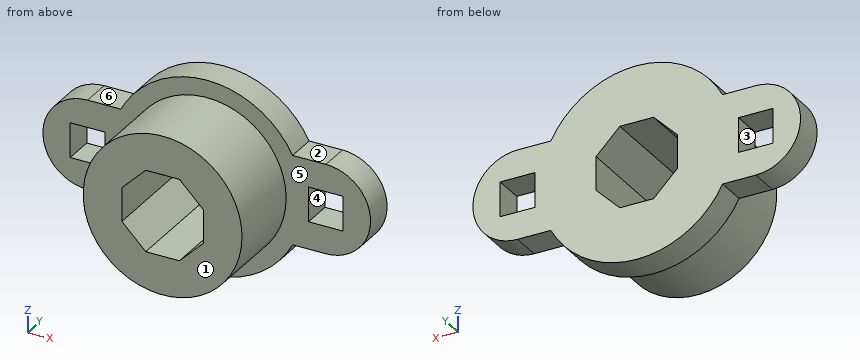
from build123d import *

# Parameters (mm, degrees)
SKETCH1_R           = 8
BOSS_EXTRUDE1_DEPTH = 8
SKETCH2_R           = 9.75
BOSS_EXTRUDE2_DEPTH = 3
BOSS_EXTRUDE3_DEPTH = 3
CUT_EXTRUDE2_REACH  = 13
SKETCH5_W           = 3.5
SKETCH5_H           = 3.5
CUT_EXTRUDE1_DEPTH  = 12


with BuildPart() as part:
    # Sketch1 → Boss-Extrude1 (new body)
    with BuildSketch(Plane(origin=(0, 0, 0), x_dir=(1, 0, 0), z_dir=(0, 1, 0))):
        Circle(SKETCH1_R)
    extrude(amount=BOSS_EXTRUDE1_DEPTH)

    # Sketch2 → Boss-Extrude2 (add)
    with BuildSketch(Plane(origin=(0, 8, 0), x_dir=(1, 0, 0), z_dir=(0, 1, 0))):
        Circle(SKETCH2_R)
    extrude(amount=BOSS_EXTRUDE2_DEPTH)

    # Sketch4 → Boss-Extrude3 (add)
    with BuildSketch(Plane(origin=(0, 11, 0), x_dir=(1, 0, 0), z_dir=(0, 1, 0))):
        with BuildLine():
            Line((12, -4.5), (-12, -4.5))
            ThreePointArc((-12, -4.5), (-16.5, 0), (-12, 4.5))
            Line((-12, 4.5), (12, 4.5))
            ThreePointArc((12, 4.5), (16.5, 0), (12, -4.5))
        make_face()
    extrude(amount=-BOSS_EXTRUDE3_DEPTH)

    # Sketch5 → Cut-Extrude2 (cut, up to next)
    with BuildSketch(Plane(origin=(0, 11, 0), x_dir=(1, 0, 0), z_dir=(0, 1, 0)), mode=Mode.PRIVATE) as cut_extrude2_sk1:
        with Locations((-12, 0)):
            Rectangle(SKETCH5_W, SKETCH5_H)
    cut_extrude2_tool1 = extrude(cut_extrude2_sk1.sketch, amount=-CUT_EXTRUDE2_REACH, mode=Mode.PRIVATE) & part.part
    add(cut_extrude2_tool1.solids().sort_by_distance((-12, 11, 0))[0], mode=Mode.SUBTRACT)
    # Sketch5 → Cut-Extrude2 (cut, up to next)
    with BuildSketch(Plane(origin=(0, 11, 0), x_dir=(1, 0, 0), z_dir=(0, 1, 0)), mode=Mode.PRIVATE) as cut_extrude2_sk2:
        with Locations((12, 0)):
            Rectangle(SKETCH5_W, SKETCH5_H)
    cut_extrude2_tool2 = extrude(cut_extrude2_sk2.sketch, amount=-CUT_EXTRUDE2_REACH, mode=Mode.PRIVATE) & part.part
    add(cut_extrude2_tool2.solids().sort_by_distance((12, 11, 0))[0], mode=Mode.SUBTRACT)

    # Sketch3 → Cut-Extrude1 (cut, through all)
    with BuildSketch(Plane(origin=(0, 11, 0), x_dir=(1, 0, 0), z_dir=(0, 1, 0))):
        Polygon((4.1, 1.698275606), (1.698275606, 4.1), (-1.698275606, 4.1), (-4.1, 1.698275606), (-4.1, -1.698275606), (-1.698275606, -4.1), (1.698275606, -4.1), (4.1, -1.698275606), align=None)
    extrude(amount=-CUT_EXTRUDE1_DEPTH, mode=Mode.SUBTRACT)


solid = part.part
The listing builds one solid part. Answer for the finished solid, in the listing's coordinates (mm). Face numbers are marked on the shaded views. A direction names the side the tool comes from. Round coordinates to 2 decimals unless told otherwise and drop trailing zeros. Order: outer loops, then holes, each group sorted by start corner. A loop starts at its lowest first (then second) coordinate and runs counter-clockwise, first axis right, second up. Notation, with made-up numbers: (54.5, 74) -> (77.5, 74) arc R29 cw to (77.5, 111) -> close; hole circle Ø11 at (26.25, 44.5). An arc over 180 degrees is marked (long way). Write each question's results on one line, items separated by ' | '. Start each with the question number.
Q1. Which of the six approach directions +Z, -Z, +X, -X, +Y, -Y give full straight-line access (tool end or side, diameter ignored) to the marked faces 4, 5 and 6?
Q2. The mould has two halves that part along Z. Classify the marked faces 1, 2 and 3: pulls with the +Z half, pulls with the -Z half, needs draft (parallel to the pull), parting line crosses it, or undercut.
Q3. Find section A-A (y = 2.75). Determine the outline of the cut face in (x, z), then the cut area to 3 significant figures.
Q4. Straight lines are drawn through the part: probe 1 along Z at (x, y) = (-3, 6); probe 2 along Y at (x, z) = (14, 4); probe 3 along X at (y, z) = (0.5, 1.5). For each, find the intervals that lie inside material, in ascending order. Write a range as from..to.
Q5. Find section C-C (y = 10). Determine the outline of the cut face in (x, z).
Q6. Find section B-B (x = 0). Determine the outline of the cut face in (y, z), then the cut area to 3 significant figures.
Q7. Each of these flat-tipped pins is pushed along its axis until it touches: pin 1 (1.7 mm diameter, centred on y = 3.5, z = -0.5, fed in from -X); pin 2 (2.5 mm diameter, centred on x = 13, y = 9.5, fed in from +Z); pin 3 (1 mm diameter, centred on x = 7, y = 5, fed in from -Z). Where does it stop, or does it pass through?
Q8. Find section D-D (z = 5.25). Determine the outline of the cut face in (x, y), then the cut area to 3 significant figures.
Worked answers:
1) face 4: +Y, -Y | face 5: -Y | face 6: +Z, -X, +Y, -Y
2) face 1: needs draft | face 2: pulls with the +Z half | face 3: undercut
3) outline: circle Ø16 at (0, 0); hole (-4.1, -1.7) -> (-1.7, -4.1) -> (1.7, -4.1) -> (4.1, -1.7) -> (4.1, 1.7) -> (1.7, 4.1) -> (-1.7, 4.1) -> (-4.1, 1.7) -> close | area: 145 mm2
4) probe 1: z = -7.42..-2.8, 2.8..7.42 | probe 2: y = 8..11 | probe 3: x = -7.86..-4.1, 4.1..7.86
5) outline: (-12, -4.5) -> (-8.65, -4.5) arc R9.75 ccw to (8.65, -4.5) -> (12, -4.5) arc R4.5 ccw to (12, 4.5) -> (8.65, 4.5) arc R9.75 ccw to (-8.65, 4.5) -> (-12, 4.5) arc R4.5 ccw to start; hole (-13.75, -1.75) -> (-10.25, -1.75) -> (-10.25, 1.75) -> (-13.75, 1.75) -> close; hole (-4.1, -1.7) -> (-1.7, -4.1) -> (1.7, -4.1) -> (4.1, -1.7) -> (4.1, 1.7) -> (1.7, 4.1) -> (-1.7, 4.1) -> (-4.1, 1.7) -> close; hole (10.25, -1.75) -> (13.75, -1.75) -> (13.75, 1.75) -> (10.25, 1.75) -> close
6) outline: (0, -8) -> (8, -8) -> (8, -9.75) -> (11, -9.75) -> (11, -4.1) -> (0, -4.1) -> close; (0, 4.1) -> (11, 4.1) -> (11, 9.75) -> (8, 9.75) -> (8, 8) -> (0, 8) -> close | area: 96.3 mm2
7) pin 1: stops at x = -8 | pin 2: stops at z = 4.5 | pin 3: stops at z = -4.66
8) outline: (-8.22, 8) -> (-6.04, 8) -> (-6.04, 0) -> (6.04, 0) -> (6.04, 8) -> (8.22, 8) -> (8.22, 11) -> (-8.22, 11) -> close | area: 146 mm2
